Check sheet for the modelled part. Datum: model origin and axes. Units: mm. Round coordinates to 2 decimals unless told otherwise and drop trailing zeros. Loops run counter-clockwise (first coordinate to the right, second up) from the corner with the lowest first, then second, coordinate; pieces in that order, holes last. Notation, with made-up numbers: (86, -18) -> (108, -18) arc R16 ccw to (108, 6) -> close; hole circle Ø11 at (32, 17.5). An arc over 180 degrees is marked (long way). Return JSON: item names as keys, results as strings.
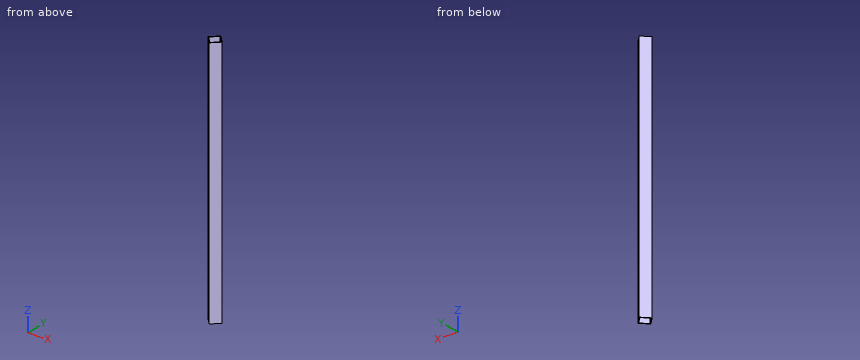
from build123d import *

# Parameters (mm, degrees)
EXTRUDE_1_DEPTH     = 610
SKETCH_2_R          = 2.75
CUT_EXTRUDE_1_DEPTH = 38.499979182


with BuildPart() as part:
    # 草圖1 → 填料-伸長1 (new body)
    with BuildSketch(Plane.XY):
        Polygon((0, 0), (17.69379362, -17.661530719), (0.032262901, -35.355324339), (-17.661530719, -17.69379362), align=None)
        Polygon((0.001935774, -2.12131946), (-15.540211259, -17.691857846), (0.030327127, -33.234004879), (15.57247416, -17.663466493), align=None, mode=Mode.SUBTRACT)
    extrude(amount=EXTRUDE_1_DEPTH)

    # 草圖2 → 除料-伸長1 (cut, through all)
    with BuildSketch(Plane(origin=(0, 0, 0), x_dir=(0.707751745, -0.706461229, 0), z_dir=(0.706461229, 0.707751745, 0))):
        with Locations((12.5, -463)):
            Circle(SKETCH_2_R)
        with Locations((12.5, -507)):
            Circle(SKETCH_2_R)
        with Locations((12.5, -103)):
            Circle(SKETCH_2_R)
        with Locations((12.5, -147)):
            Circle(SKETCH_2_R)
    extrude(amount=-CUT_EXTRUDE_1_DEPTH, mode=Mode.SUBTRACT)


solid = part.part
Q1. Section check A-A (z = 448.5). Record the boundary of the cut face in (x, y), then the cut area to 3 significant figures.
Results list:
{"outline": "(-17.66, -17.69) -> (0.03, -35.36) -> (17.69, -17.66) -> (0, 0) -> close; hole (-15.54, -17.69) -> (0.03, -33.23) -> (15.57, -17.66) -> (0, -2.12) -> close", "area": "141 mm^2"}
Q2. Material ranges on line 1 (Y direction, x = 0, z = 530); line 2 (Z direction, x = 6.5, y = -7.5); line 3 (Y direction, x = 6.5, z = 263), recorded low to high.
Results list:
{"line 1": "-35.32 to -33.2, -2.12 to 0", "line 2": "0 to 102.11, 103.89 to 146.11, 147.89 to 462.11, 463.89 to 506.11, 507.89 to 610", "line 3": "-28.88 to -26.75, -8.61 to -6.49"}
Q3. Go/stop test with flat-tipped pins: pin 1 (10 mm diameter, centred on x = 8, y = -18, fed in from -Z); pin 2 (10 mm diameter, centred on y = -28.5, z = 377, fed in from +X); pin 3 (2 mm diameter, centred on y = -27, z = 459.5, fed in from +X). Record where each tip stops, or that it passes through.
Results list:
{"pin 1": "through", "pin 2": "x = 11.87", "pin 3": "x = 9.37"}
